Read the model definition and answer for the solid it produces. Units are mm, in the model's axes. Round coordinates to 2 decimals unless told otherwise and drop trailing zeros. One line per item, written item: value. Start each with the question number.
(1) A cutting plane is placed at A-A, the plane z = 1.15. State how many separate pieces and enclosed holes the cut face has, plus the area to 3 significant figures.
(2) Find the intervals of material crossed by L1, parallel to Y at x = 8, z = 1.55; L2, parallel to Y at x = 25, z = 0.6; L3, parallel to X at y = 3.5, z = 0.5, in increasing order.
(3) The mould has two halves that part along X. Classify faces 1 (the face through (-36.03, -0.91, 1.57)), 2 (the face through (9, 2, 0)), 3 (the face through (-46.275, -4.399, 1.61)): +X half, -X half, draft (parallel to the pull), parting line (faces both ways), or undercut.
from build123d import *

# Parameters (mm, degrees)
F0_W     = 112.6090909091
F0_H     = 10
F0_R     = 1.5
F1_DEPTH = 3.175
F2_R     = 2


# Not quite as in the source:
# - a length typed as a fraction of an inch, garbled in the dataset ("3 / 203.2 mm" for 3/8 in), is restored


with BuildPart() as f1:
    # F0 (on Top) → F1 (new body)
    with BuildSketch(Plane.XY):
        with Locations((9.4590909091, 0)):
            Rectangle(F0_W, F0_H)
        with Locations((-43.5454545455, 0)):
            Circle(F0_R, mode=Mode.SUBTRACT)
        with Locations((-34.8363636364, 0)):
            Circle(F0_R, mode=Mode.SUBTRACT)
        with Locations((-26.1272727273, 0)):
            Circle(F0_R, mode=Mode.SUBTRACT)
        with Locations((-17.4181818182, 0)):
            Circle(F0_R, mode=Mode.SUBTRACT)
        with Locations((-8.7090909091, 0)):
            Circle(F0_R, mode=Mode.SUBTRACT)
        with Locations((-0.0571461482, 0)):
            Circle(F0_R, mode=Mode.SUBTRACT)
        with Locations((8.7090909091, 0)):
            Circle(F0_R, mode=Mode.SUBTRACT)
        with Locations((17.4181818182, 0)):
            Circle(F0_R, mode=Mode.SUBTRACT)
        with Locations((26.1272727273, 0)):
            Circle(F0_R, mode=Mode.SUBTRACT)
        with Locations((34.8363636364, 0)):
            Circle(F0_R, mode=Mode.SUBTRACT)
        with Locations((43.5454545455, 0)):
            Circle(F0_R, mode=Mode.SUBTRACT)
        with Locations((52.2545454545, 0)):
            Circle(F0_R, mode=Mode.SUBTRACT)
        with Locations((60.9636363636, 0)):
            Circle(F0_R, mode=Mode.SUBTRACT)
    extrude(amount=F1_DEPTH)

    # F2
    f2_edges = [f1.edges().sort_by_distance(p)[0] for p in [
        (-46.845455, 5, 1.5875),
        (-46.845455, -5, 1.5875),
        (65.763636, 5, 1.5875),
        (65.763636, -5, 1.5875),
    ]]
    fillet(f2_edges, radius=F2_R)


solid = f1.part
Here are the results:
1. separate pieces: 1
1. enclosed holes: 13
1. area: 1,030 mm²
2. L1: -5 to -1.32, 1.32 to 5
2. L2: -5 to -0.99, 0.99 to 5
2. L3: -46.78 to 65.7
3. face 1: undercut
3. face 2: draft
3. face 3: -X half
